```python
from build123d import *

# Parameters (mm, degrees)
F0_W     = 231.775
F0_H     = 79.375
F1_DEPTH = 25.4
F3_DEPTH = 3.175


with BuildPart() as f1:
    # F0 (on Top) → F1 (new body)
    with BuildSketch(Plane.XY):
        Rectangle(F0_W, F0_H)
    extrude(amount=F1_DEPTH)

    # F2 (on face) → F3 (cut)
    with BuildSketch(Plane.XY.offset(25.4)):
        Polygon((63.5, 16.328571), (-88.9, 0), (63.5, -16.328571), (88.9, 0), align=None)
    extrude(amount=-F3_DEPTH, mode=Mode.SUBTRACT)


solid = f1.part
```
The model under review builds one solid part; all positions refer to its coordinate system, in mm. A direction names the side the tool comes from. Coordinates: 2 decimals unless noted, no trailing zeros. Loops run counter-clockwise (first coordinate to the right, second up) from the corner with the lowest first, then second, coordinate; pieces in that order, holes last. Notation, with made-up numbers: (72.25, 21) -> (98.25, 21) arc R10 cw to (98.25, 36) -> close; hole circle Ø7 at (30, 10). An arc over 180 degrees is marked (long way). Answer as CSV lines item,"result".
Item 1: For L1, parallel to Y at x = -66, z = 24; L2, parallel to Y at x = -82.5, z = 24, list the stretches that pass through material, from the lowest coordinate up.
Results below:
L1,"y = -39.69 to -2.45, 2.45 to 39.69"
L2,"y = -39.69 to -0.69, 0.69 to 39.69"
Item 2: Machinability: for faces 5 (the flat face through (115.888, -1, 13)), 6 (the flat face through (76.02, -8.28, 23.83)), which of the approach directions +Z, -Z, +X, -X, +Y, -Y give a long, thin tool a straight path to every point of the face, cutting with its end or side? Answer none if there is none.
Results below:
face 5,"+Z, -Z, +X, +Y, -Y"
face 6,"+Z"
Item 3: Take a section at B-B, the plane y = -4. State the section outline as (x, z) points (1 decimal).
Results below:
outline,"(-115.9, 0) -> (115.9, 0) -> (115.9, 25.4) -> (82.7, 25.4) -> (82.7, 22.2) -> (-51.6, 22.2) -> (-51.6, 25.4) -> (-115.9, 25.4) -> close"
Item 4: Draft analysis for pull direction X (two halves, no side actions). For faces 1 (the flat face through (-115.888, -1, 13)), 2 (the flat face through (-2, 39.688, 13)), 3 (the flat face through (-11.63, 8.28, 23.83)), 4 (the flat face through (-13.77, -8.05, 23.83)), state which applies: +X half, -X half, draft (parallel to the pull), parting line (faces both ways), or undercut.
Results below:
face 1,"-X half"
face 2,"draft"
face 3,"undercut"
face 4,"undercut"
Item 5: Take a section at A-A, the plane x = 75. State the section outline as (y, z) points (1 decimal).
Results below:
outline,"(-39.7, 0) -> (39.7, 0) -> (39.7, 25.4) -> (8.9, 25.4) -> (8.9, 22.2) -> (-8.9, 22.2) -> (-8.9, 25.4) -> (-39.7, 25.4) -> close"
